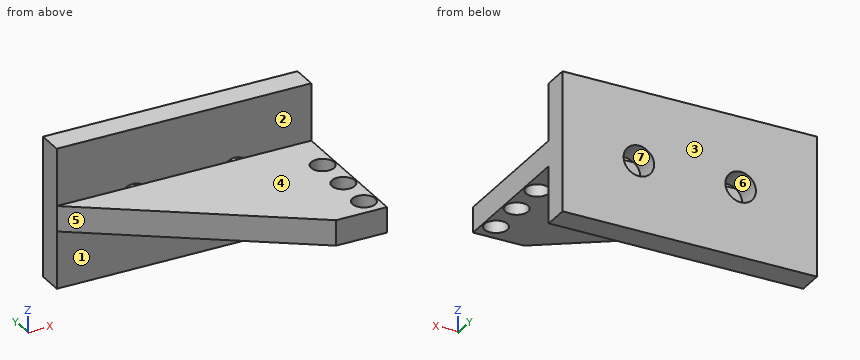
from build123d import *

# Parameters (mm, degrees)
SKETCH1_W           = 20
SKETCH1_H           = 11
BOSS_EXTRUDE1_DEPTH = 2
BOSS_EXTRUDE2_DEPTH = 2
SKETCH3_R           = 0.9
CUT_EXTRUDE1_DEPTH  = 2
SKETCH4_R           = 1.2
CUT_EXTRUDE2_DEPTH  = 2


with BuildPart() as part:
    # Sketch1 → Boss-Extrude1 (new body)
    with BuildSketch(Plane(origin=(0, 0, 0), x_dir=(1, 0, 0), z_dir=(0, 1, 0))):
        with Locations((-10, 0)):
            Rectangle(SKETCH1_W, SKETCH1_H)
    extrude(amount=-BOSS_EXTRUDE1_DEPTH)

    # Sketch2 → Boss-Extrude2 (add)
    with BuildSketch(Plane.XY.offset(-1)):
        Polygon((0, 0), (0, -13), (-4, -13), (-20, -2), (-20, 0), align=None)
    extrude(amount=BOSS_EXTRUDE2_DEPTH)

    # Sketch3 → Cut-Extrude1 (cut)
    with BuildSketch(Plane.XY.offset(-1)):
        with Locations((-1, -5.5)):
            Circle(SKETCH3_R)
        with Locations((-1, -8.5)):
            Circle(SKETCH3_R)
        with Locations((-1, -11.5)):
            Circle(SKETCH3_R)
    extrude(amount=CUT_EXTRUDE1_DEPTH, mode=Mode.SUBTRACT)

    # Sketch4 → Cut-Extrude2 (cut)
    with BuildSketch(Plane(origin=(0, 0, 0), x_dir=(1, 0, 0), z_dir=(0, 1, 0))):
        with Locations(Location((-6, 0, 0), (0, 0, 270))):
            Circle(SKETCH4_R)
        with Locations(Location((-14, 0, 0), (0, 0, 270))):
            Circle(SKETCH4_R)
    extrude(amount=-CUT_EXTRUDE2_DEPTH, mode=Mode.SUBTRACT)


solid = part.part
Model file for the job. Use its own axes, mm. Face numbers are marked on the shaded views. A direction names the side the tool comes from. Give positions to 0.01 mm unless a question says otherwise; leave off trailing zeros. Loops run counter-clockwise (first coordinate to the right, second up) from the corner with the lowest first, then second, coordinate; pieces in that order, holes last.
1) Pull direction Z, two halves, no side cores. Call the marked faces 4, 5, 6 and 7: +Z half, -Z half, draft (parallel to the pull), parting line (faces both ways), or undercut.
2) Wall check: line 1 (Y direction, x = -1, z = 0.4); line 2 (X direction, y = -0.45, z = 0); line 3 (Z direction, x = -6, y = -0.75). Give the ranges that are in metal, low to high.
3) Saw through at D-D (x = -6). Write the cut outline in (y, z) (3 decimals).
4) Saw through at C-C (y = -8.5). Write the cut outline in (x, z).
5) Tool access for the marked faces 1, 2 and 3: list every direction of +Z, -Z, +X, -X, +Y, -Y with a clear straight run to the whole face (end or side of a thin tool).
6) Saw through at B-B (z = 0). Write the cut outline in (x, y), plus the area to 3 significant figures.
7) Saw through at A-A (x = -1). Write the cut outline in (y, z).
8) Flat gauge pins, fed straight in: pin 1 Ø3.5 at (x, y) = (-8.5, -10) entering from -Z; pin 2 Ø1 at (x, z) = (-3.5, 4.5) entering from -Y; pin 3 Ø2 at (x, z) = (-5.5, 0.5) entering from +Y; pin 4 Ø3 at (x, y) = (-12, -4) entering from +Z. Where does each tip first touch, or does it go through?
Answer block:
1. face 4: +Z half
1. face 5: draft
1. face 6: undercut
1. face 7: undercut
2. line 1: y = -13 to -12.4, -10.6 to -9.4, -7.6 to -6.4, -4.6 to 0
2. line 2: x = -20 to -15.2, -12.8 to -7.2, -4.8 to 0
2. line 3: z = -5.5 to -1.2, 1.2 to 5.5
3. outline: (-11.625, -1) - (-2, -1) - (-2, 1) - (-11.625, 1) - close; (-2, -5.5) - (0, -5.5) - (0, -1.2) - (-2, -1.2) - close; (-2, 1.2) - (0, 1.2) - (0, 5.5) - (-2, 5.5) - close
4. outline: (-10.55, -1) - (-1.9, -1) - (-1.9, 1) - (-10.55, 1) - close; (-0.1, -1) - (0, -1) - (0, 1) - (-0.1, 1) - close
5. face 1: -Z, +X, -X, -Y
5. face 2: +Z, +X, -X, -Y
5. face 3: +Z, -Z, +X, -X, +Y
6. outline: (-20, -2) - (-4, -13) - (0, -13) - (0, 0) - (-4.8, 0) - (-4.8, -2) - (-7.2, -2) - (-7.2, 0) - (-12.8, 0) - (-12.8, -2) - (-15.2, -2) - (-15.2, 0) - (-20, 0) - close; hole circle Ø1.8 at (-1, -11.5); hole circle Ø1.8 at (-1, -8.5); hole circle Ø1.8 at (-1, -5.5)
6. area: 155 mm2
7. outline: (-13, -1) - (-12.4, -1) - (-12.4, 1) - (-13, 1) - close; (-10.6, -1) - (-9.4, -1) - (-9.4, 1) - (-10.6, 1) - close; (-7.6, -1) - (-6.4, -1) - (-6.4, 1) - (-7.6, 1) - close; (-4.6, -1) - (-2, -1) - (-2, -5.5) - (0, -5.5) - (0, 5.5) - (-2, 5.5) - (-2, 1) - (-4.6, 1) - close
8. pin 1: stops at z = -1
8. pin 2: stops at y = -2
8. pin 3: stops at y = 0
8. pin 4: stops at z = 1
